from build123d import *

# Parameters (mm, degrees)
SKETCH1_W             = 37
SKETCH1_H             = 85
BOSS_EXTRUDE1_DEPTH   = 686
BOSS_EXTRUDE1_2_DEPTH = 686
SKETCH2_W             = 38
SKETCH2_H             = 85
BOSS_EXTRUDE2_DEPTH   = 610


with BuildPart() as part:
    # Sketch1 → Boss-Extrude1 (new body)
    with BuildSketch(Plane.XY):
        with Locations((18.5, 42.5)):
            Rectangle(SKETCH1_W, SKETCH1_H)
    extrude(amount=BOSS_EXTRUDE1_DEPTH)



with BuildPart() as body_2:
    # Sketch1 → Boss-Extrude1 2 (new body)
    with BuildSketch(Plane.XY):
        with Locations((-628.5, 42.5)):
            Rectangle(SKETCH1_W, SKETCH1_H)
    extrude(amount=BOSS_EXTRUDE1_2_DEPTH)


with BuildPart() as part_1:
    add(part.part)

    add(body_2.part)  # Boss-Extrude2 merges body 2
    # Sketch2 → Boss-Extrude2 (add)
    with BuildSketch(Plane(origin=(-610, 0, 0), x_dir=(0, 0, -1), z_dir=(1, 0, 0))):
        with Locations((-667, 42.5)):
            Rectangle(SKETCH2_W, SKETCH2_H)
        with Locations((-19, 42.5)):
            Rectangle(SKETCH2_W, SKETCH2_H)
    extrude(amount=BOSS_EXTRUDE2_DEPTH)


solid = part_1.part
Verification items for the finished model (mm, model axes). A direction names the side the tool comes from. Round coordinates to 2 decimals unless told otherwise and drop trailing zeros. Loops run counter-clockwise (first coordinate to the right, second up) from the corner with the lowest first, then second, coordinate; pieces in that order, holes last. Notation, with made-up numbers: (78.5, -10.5) - (126.5, -10.5) arc R14 ccw to (126.5, 11.5) - close; hole circle Ø2 at (-34, 44). An arc over 180 degrees is marked (long way). Answer in a Markdown table with one row per item. Add a question column.
Q1. Release check for a two-part mould opening along Z. For faces 1 (the face through (-310, 42, 686)), 2 (the face through (-610, 42, 339)), 3 (the face through (-357, 85, 649)) record: pulls with the +Z half, pulls with the -Z half, needs draft (parallel to the pull), parting line crosses it, or undercut.
Q2. Material ranges on line 1 (Z direction, x = -232, y = 47); line 2 (X direction, y = 25, z = 397), recorded low to high.
Q3. Tool access check on faces 4 (the face through (-309, 42, 648)), 5 (the face through (-647, 42, 338)). Record the directions out of +Z, -Z, +X, -X, +Y, -Y that give a thin tool (end or side, any length) a straight path to the whole face; none if there is none.
Q4. Section check C-C on x = -530. Enter the section's corners in (y, z).
Q5. Section check B-B on y = 73. Enter the section's corners in (x, z), plus the area to 3 significant figures.
Q6. Section check A-A on z = 396. Enter the section's corners in (x, y), plus the area to 3 significant figures.
Found:
| question | item | result |
|---|---|---|
| 1 | face 1 | pulls with the +Z half |
| 1 | face 2 | undercut |
| 1 | face 3 | needs draft |
| 2 | line 1 | z = 0 to 38, 648 to 686 |
| 2 | line 2 | x = -647 to -610, 0 to 37 |
| 3 | face 4 | +Y, -Y |
| 3 | face 5 | +Z, -Z, -X, +Y, -Y |
| 4 | outline | (0, 0) - (85, 0) - (85, 38) - (0, 38) - close; (0, 648) - (85, 648) - (85, 686) - (0, 686) - close |
| 5 | outline | (-647, 0) - (37, 0) - (37, 686) - (-647, 686) - close; hole (-610, 38) - (0, 38) - (0, 648) - (-610, 648) - close |
| 5 | area | 97,100 mm² |
| 6 | outline | (-647, 0) - (-610, 0) - (-610, 85) - (-647, 85) - close; (0, 0) - (37, 0) - (37, 85) - (0, 85) - close |
| 6 | area | 6,290 mm² |
